```python
from build123d import *

# Parameters (mm, degrees)
EXTRUDE_1_DEPTH     = 0.25
EXTRUDE_1_2_DEPTH   = 0.25
CUT_EXTRUDE_START   = -0.8
CUT_EXTRUDE_1_DEPTH = 0.8


with BuildPart() as part:
    # Sketch 1 → Extrude 1 (new, symmetric)
    with BuildSketch(Plane.XZ):
        Polygon((-1.52, 3.6), (-1.52, 1), (-1.62, 1), (-1.62, 0), (-1.52, 0), (-1.52, -3), (-1.02, -3), (-1.02, 0), (-0.92, 0), (-0.92, 1), (-1.02, 1), (-1.02, 3.6), align=None)
    extrude(amount=EXTRUDE_1_DEPTH, both=True)



with BuildPart() as body_2:
    # Sketch 1 → Extrude 1 2 (new, symmetric)
    with BuildSketch(Plane.XZ):
        Polygon((1.02, 3.6), (1.02, 1), (0.92, 1), (0.92, 0), (1.02, 0), (1.02, -3), (1.52, -3), (1.52, 0), (1.62, 0), (1.62, 1), (1.52, 1), (1.52, 3.6), align=None)
    extrude(amount=EXTRUDE_1_2_DEPTH, both=True)


with BuildPart() as part_1:
    add(part.part)

    add(body_2.part)  # Revolve 1 merges body 2
    # Sketch 2 → Revolve 1 (revolve)
    with BuildSketch(Plane(origin=(0, 0, 0), x_dir=(1, 0, 0), z_dir=(0, 1, 0))):
        with BuildLine():
            Line((0, -3.6), (0, -8.9))
            ThreePointArc((0, -8.9), (1.060660172, -8.460660172), (1.5, -7.4))
            Line((1.5, -7.4), (1.5, -4.4))
            Line((1.5, -4.4), (1.95, -4.4))
            Line((1.95, -4.4), (1.95, -3.6))
            Line((1.95, -3.6), (0, -3.6))
        make_face()
    revolve(axis=Axis((0, 0, 3.6), (0, 0, -1)))

    # Sketch 3 → Cut-Extrude 1 (cut)
    with BuildSketch(Plane.XY.offset(4.4).offset(CUT_EXTRUDE_START)):
        with BuildLine():
            Line((1.5, 1.245993579), (1.5, -1.245993579))
            ThreePointArc((1.5, -1.245993579), (1.95, 0), (1.5, 1.245993579))
        make_face()
    extrude(amount=CUT_EXTRUDE_1_DEPTH, mode=Mode.SUBTRACT)


solid = part_1.part
```
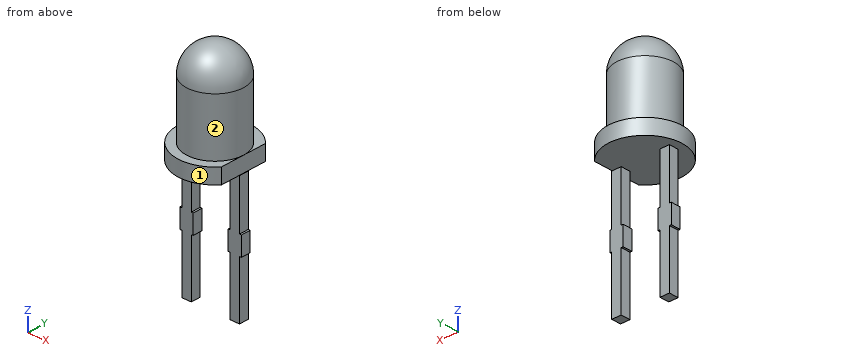
CAD build for the part. Positions are in the model's coordinates, mm. Face numbers are marked on the shaded views. A direction names the side the tool comes from. Round coordinates to 2 decimals unless told otherwise and drop trailing zeros. Order: outer loops, then holes, each group sorted by start corner. A loop starts at its lowest first (then second) coordinate and runs counter-clockwise, first axis right, second up. Notation, with made-up numbers: (80, 18.5) - (102, 18.5) arc R17 ccw to (102, 50.5) - close; hole circle Ø3 at (82, 42). An arc over 180 degrees is marked (long way). Answer in a Markdown table with one row per item. Add a question column.
(1) Band-saw the part on C-C on y = -0.95. List the corners of the cut face in (x, z).
(2) 3-axis set-ups, long thin cutter, end or side, ignore diameter. For the marked faces 1 and 2: which of +Z, -Z, +X, -X, +Y, -Y reach the whole face in a straight line?
(3) Drop flat-ended pins along their axis: pin 1 Ø0.6 at (x, z) = (1, -0.5) entering from +Y; pin 2 Ø0.6 at (y, z) = (0, 2) entering from +X; pin 3 Ø1 at (x, z) = (1, 6) entering from +Y. Give the stop position or say it passes through.
(4) Band-saw the part on B-B on x = 0.15. List the corners of the cut face in (y, z), and give its area (3 significant figures).
(5) Band-saw the part on A-A on z = 3. List the corners of the cut face in (x, y).
(6) Probe L1, parallel to X at y = 0.15, z = 2.25; L2, parallel to X at y = 1.1, z = 5.5; L3, parallel to Z at x = -0.5, y = -1.65. List the from-to ranges inside material, lowest first. Write a range as [from, to].
(7) Band-saw the part on D-D on z = 6. List the corners of the cut face in (x, y), and give its area (3 significant figures).
Data:
| question | item | result |
|---|---|---|
| 1 | outline | (-1.7, 3.6) - (1.5, 3.6) - (1.5, 4.4) - (1.16, 4.4) - (1.16, 7.4) arc R1.16 ccw to (-1.16, 7.4) - (-1.16, 4.4) - (-1.7, 4.4) - close |
| 2 | face 1 | +Z, -Z |
| 2 | face 2 | +Z |
| 3 | pin 1 | stops at y = 0.25 |
| 3 | pin 2 | stops at x = 1.52 |
| 3 | pin 3 | stops at y = 1.41 |
| 4 | outline | (-1.94, 3.6) - (1.94, 3.6) - (1.94, 4.4) - (1.49, 4.4) - (1.49, 7.4) arc R1.49 ccw to (-1.49, 7.4) - (-1.49, 4.4) - (-1.94, 4.4) - close |
| 4 | area | 15.6 mm^2 |
| 5 | outline | (-1.52, -0.25) - (-1.02, -0.25) - (-1.02, 0.25) - (-1.52, 0.25) - close; (1.02, -0.25) - (1.52, -0.25) - (1.52, 0.25) - (1.02, 0.25) - close |
| 6 | L1 | x = [-1.52, -1.02], [1.02, 1.52] |
| 6 | L2 | x = [-1.02, 1.02] |
| 6 | L3 | z = [3.6, 4.4] |
| 7 | outline | circle Ø3 at (0, 0) |
| 7 | area | 7.07 mm^2 |
